Read the model definition and answer for the solid it produces. Units are mm, in the model's axes. A direction names the side the tool comes from. Coordinates: 2 decimals unless noted, no trailing zeros. Write each loop counter-clockwise with the first axis right and the second up, starting at its lowest first coordinate (ties: lowest second). Pieces come first, ordered by that corner, then holes.
1) Find the intervals of material crossed by line 1 (X direction, y = 8.25, z = 1.9); line 2 (X direction, y = 9.25, z = 0.6); line 3 (Y direction, x = -5, z = 3), in increasing order.
2) Which of the six approach directions +Z, -Z, +X, -X, +Y, -Y give full straight-line access (tool end or side, diameter ignored) to faces 5 (the face through (-2.423, -1, 2)), 6 (the face through (-12, 17, 2)), 7 (the face through (-9.423, -1, 3)), 8 (the face through (-27.173, 3, 2))?
3) Each of these flat-tipped pins is pushed along its axis until it touches: pin 1 Ø1.2 at (y, z) = (5.5, 2) entering from +X; pin 2 Ø2 at (y, z) = (-2, 1.5) entering from +X; pin 3 Ø10.5 at (x, y) = (-14.5, -3) entering from +Z; pin 4 Ø2 at (x, y) = (5, 15.97) entering from -Z. Where does it stop, or does it pass through?
4) The part is cut by section C-C (z = 0.8). Determine the outline of the cut face in (x, y).
5) Determine the mould class of faces 1 (the face through (12, 12, 2)), 2 (the face through (0, 19.974, 2)), 3 (the face through (-16, 6.204, 3)), 4 (the face through (-6.384, -3.295, 1.972)) for opening direction Y: +Y half, -Y half, draft (parallel to the pull), parting line (faces both ways), or undercut.
6) The part is cut by section B-B (y = -1). Determine the outline of the cut face in (x, z), then the cut area to 3 significant figures.
7) The part is cut by section D-D (x = -18.5). Determine the outline of the cut face in (y, z).
8) The part is cut by section A-A (x = 5). Determine the outline of the cut face in (y, z), then the cut area to 3 significant figures.
from build123d import *

# Parameters (mm, degrees)
SKETCH1_R           = 1.85
BOSS_EXTRUDE1_DEPTH = 4
FILLET1_R           = 2.5
SKETCH2_W           = 13
SKETCH2_H           = 20
CUT_EXTRUDE1_DEPTH  = 2
FILLET2_R           = 2


with BuildPart() as part:
    # Sketch1 → Boss-Extrude1 (new body)
    with BuildSketch(Plane.XY):
        Polygon((-12, 19.974398687), (12, 19.974398687), (12, 4.787936134), (-2.422914658, 4.787936134), (-2.422914658, -6.752077686), (-29.422914658, -6.752077686), (-29.422914658, 13.7384821), (-12, 13.7384821), align=None)
        with Locations((-5, 15.974398687)):
            Circle(SKETCH1_R, mode=Mode.SUBTRACT)
        with Locations((5, 15.974398687)):
            Circle(SKETCH1_R, mode=Mode.SUBTRACT)
        with BuildLine():
            Line((-4.672914658, 8.454123535), (-4.672914658, -1.545876465))
            ThreePointArc((-4.672914658, -1.545876465), (-6.422914658, -3.295876465), (-8.172914658, -1.545876465))
            Line((-8.172914658, -1.545876465), (-8.172914658, 8.454123535))
            ThreePointArc((-8.172914658, 8.454123535), (-6.422914658, 10.204123534), (-4.672914658, 8.454123535))
        make_face(mode=Mode.SUBTRACT)
        with BuildLine():
            Line((-23.672914658, 8.454123535), (-23.672914658, -1.545876465))
            ThreePointArc((-23.672914658, -1.545876465), (-25.422914658, -3.295876465), (-27.172914658, -1.545876465))
            Line((-27.172914658, -1.545876465), (-27.172914658, 8.454123535))
            ThreePointArc((-27.172914658, 8.454123535), (-25.422914658, 10.204123534), (-23.672914658, 8.454123535))
        make_face(mode=Mode.SUBTRACT)
    extrude(amount=BOSS_EXTRUDE1_DEPTH)

    # Fillet1
    fillet1_edges = [part.edges().sort_by_distance(p)[0] for p in [
        (-12, 19.974398687, 2),
        (12, 19.974398687, 2),
        (12, 4.787936134, 2),
        (-2.422914658, 4.787936134, 2),
        (-2.422914658, -6.752077686, 2),
        (-29.422914658, -6.752077686, 2),
        (-29.422914658, 13.7384821, 2),
        (-12, 13.7384821, 2),
    ]]
    fillet(fillet1_edges, radius=FILLET1_R)

    # Sketch2 → Cut-Extrude1 (cut)
    with BuildSketch(Plane.XY.offset(4)):
        with Locations((-15.922914658, -3.795876465)):
            Rectangle(SKETCH2_W, SKETCH2_H)
    extrude(amount=-CUT_EXTRUDE1_DEPTH, mode=Mode.SUBTRACT)

    # Fillet2
    fillet2_edges = [part.edges().sort_by_distance(p)[0] for p in [
        (-9.422914658, 6.204123535, 3),
        (-22.422914658, 6.204123535, 3),
    ]]
    fillet(fillet2_edges, radius=FILLET2_R)


solid = part.part
Reported:
1. line 1: x = -29.42 to -27.17, -23.67 to -8.17, -4.67 to 12
1. line 2: x = -29.42 to -26.98, -23.86 to -7.98, -4.86 to 12
1. line 3: y = -6.75 to -2.56, 9.47 to 14.12, 17.82 to 19.97
2. face 5: +Z, -Z, +X, -Y
2. face 6: +Z, -Z, -X, +Y
2. face 7: +Z, -Y
2. face 8: +Z, -Z
3. pin 1: stops at x = 11.7
3. pin 2: stops at x = -2.42
3. pin 3: stops at z = 4
3. pin 4: passes through
4. outline: (-29.42, -4.25) arc R2.5 ccw to (-26.92, -6.75) - (-4.92, -6.75) arc R2.5 ccw to (-2.42, -4.25) - (-2.42, 2.29) arc R2.5 cw to (0.08, 4.79) - (9.5, 4.79) arc R2.5 ccw to (12, 7.29) - (12, 17.47) arc R2.5 ccw to (9.5, 19.97) - (-9.5, 19.97) arc R2.5 ccw to (-12, 17.47) - (-12, 16.24) arc R2.5 cw to (-14.5, 13.74) - (-26.92, 13.74) arc R2.5 ccw to (-29.42, 11.24) - close; hole (-27.17, -1.55) arc R1.75 ccw to (-23.67, -1.55) - (-23.67, 8.45) arc R1.75 ccw to (-27.17, 8.45) - close; hole (-8.17, -1.55) arc R1.75 ccw to (-4.67, -1.55) - (-4.67, 8.45) arc R1.75 ccw to (-8.17, 8.45) - close; hole circle Ø3.7 at (-5, 15.97); hole circle Ø3.7 at (5, 15.97)
5. face 1: draft
5. face 2: +Y half
5. face 3: -Y half
5. face 4: undercut
6. outline: (-29.42, 0) - (-27.17, 0) - (-27.17, 4) - (-29.42, 4) - close; (-23.67, 0) - (-8.17, 0) - (-8.17, 4) - (-9.42, 4) - (-9.42, 2) - (-22.42, 2) - (-22.42, 4) - (-23.67, 4) - close; (-4.67, 0) - (-2.42, 0) - (-2.42, 4) - (-4.67, 4) - close
6. area: 54.0 mm2
7. outline: (-6.75, 0) - (13.74, 0) - (13.74, 4) - (6.2, 4) - (6.2, 2) - (-6.75, 2) - close
8. outline: (4.79, 0) - (14.12, 0) - (14.12, 4) - (4.79, 4) - close; (17.82, 0) - (19.97, 0) - (19.97, 4) - (17.82, 4) - close
8. area: 45.9 mm2
